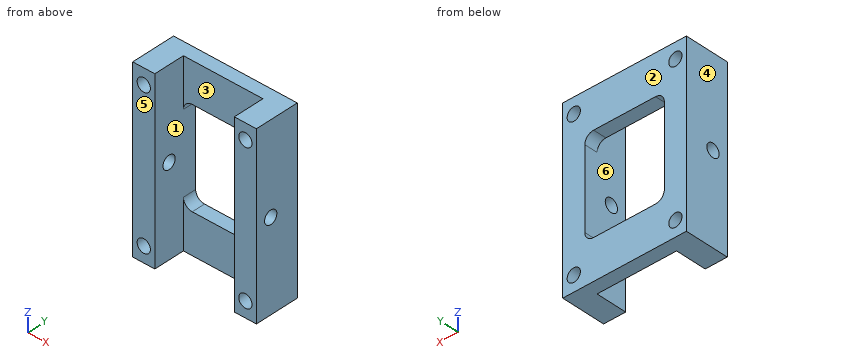
from build123d import *

# Parameters (mm, degrees)
EXTRUDE_1_DEPTH     = 40
SKETCH_2_R          = 1.5
CUT_EXTRUDE_1_DEPTH = 40
SKETCH_3_R          = 1.5
CUT_EXTRUDE_2_DEPTH = 40
SKETCH_5_W          = 18
SKETCH_5_H          = 22
CUT_EXTRUDE_3_DEPTH = 50.839743178
FILLET_3_R          = 2


with BuildPart() as part:
    # 草图1 → 凸台-拉伸1 (new body)
    with BuildSketch(Plane.XY):
        Polygon((0, 0), (0, 10), (28, 10), (28, 0), (23, 0), (23, 7), (5, 7), (5, 0), align=None)
    extrude(amount=EXTRUDE_1_DEPTH)

    # 草图2 → 切除-拉伸1 (cut)
    with BuildSketch(Plane(origin=(0, 10, 0), x_dir=(1, 0, 0), z_dir=(0, 1, 0))):
        with Locations(Location((2.5, -3.5, 0), (0, 0, 270))):
            Circle(SKETCH_2_R)
        with Locations(Location((2.5, -36.5, 0), (0, 0, 270))):
            Circle(SKETCH_2_R)
        with Locations(Location((25.5, -36.5, 0), (0, 0, 270))):
            Circle(SKETCH_2_R)
        with Locations(Location((25.5, -3.5, 0), (0, 0, 270))):
            Circle(SKETCH_2_R)
    extrude(amount=-CUT_EXTRUDE_1_DEPTH, mode=Mode.SUBTRACT)

    # 草图3 → 切除-拉伸2 (cut)
    with BuildSketch(Plane.ZY):
        with Locations((20, 3.5)):
            Circle(SKETCH_3_R)
    extrude(amount=-CUT_EXTRUDE_2_DEPTH, mode=Mode.SUBTRACT)

    # 草图5 → 切除-拉伸3 (cut, through all)
    with BuildSketch(Plane(origin=(0, 10, 0), x_dir=(1, 0, 0), z_dir=(0, 1, 0))):
        with Locations((14, -20)):
            Rectangle(SKETCH_5_W, SKETCH_5_H)
    extrude(amount=-CUT_EXTRUDE_3_DEPTH, mode=Mode.SUBTRACT)

    # 圆角3
    fillet_3_edges = [part.edges().sort_by_distance(p)[0] for p in [
        (23, 8.5, 31),
        (5, 8.5, 9),
        (5, 8.5, 31),
        (23, 8.5, 9),
    ]]
    fillet(fillet_3_edges, radius=FILLET_3_R)


solid = part.part
Verification items for the finished model (mm, model axes). Face numbers are marked on the shaded views. A direction names the side the tool comes from. Coordinates: 2 decimals unless noted, no trailing zeros. Order: outer loops, then holes, each group sorted by start corner. A loop starts at its lowest first (then second) coordinate and runs counter-clockwise, first axis right, second up. Notation, with made-up numbers: (-18.75, -38.5) -> (26.25, -38.5) arc R35 ccw to (26.25, -1.5) -> close; hole circle Ø5 at (45.25, 85). An arc over 180 degrees is marked (long way). Use CSV: the item, a comma, the result in double quotes. Start each with the question number.
Q1. Section check A-A, the plane x = 2.5. Record the cut outline in (y, z).
Q2. Draft check along X on the marked faces 4, 5 and 6. Enter one of: +X half, -X half, draft (parallel to the pull), parting line (faces both ways), or undercut.
Q3. Thickness scan on line 1 along X through (y, z) = (4.25, 3.5); line 2 along X through (y, z) = (5.75, 14); line 3 along Z through (x, y) = (14.25, 9). Record the ranges inside material, lowest first.
Q4. Section check C-C, the plane y = 3.5. Record the cut outline in (x, z), and give its area (3 significant figures).
Q5. Depth check by flat-ended pin: P1, Ø2.5, axis at x = 25.5, z = 3.5, coming from the +Y side; P2, Ø4, axis at y = 3.5, z = 20, coming from the -X side; P3, Ø5.5, axis at x = 11, z = 35.5, coming from the -Y side. Enter the tip coordinate at first touch or a pass-through.
Q6. Section check B-B, the plane y = 1.5. Record the cut outline in (x, z), and give its area (3 significant figures).
Q7. Section check D-D, the plane z = 20. Record the cut outline in (x, y), and give its area (3 significant figures).
Q8. Tool access check on the marked faces 1, 2 and 3. Record the directions out of +Z, -Z, +X, -X, +Y, -Y that give a thin tool (end or side, any length) a straight path to the whole face; none if there is none.
Returned:
1,outline,"(0, 0) -> (10, 0) -> (10, 2) -> (0, 2) -> close; (0, 5) -> (10, 5) -> (10, 35) -> (0, 35) -> close; (0, 38) -> (10, 38) -> (10, 40) -> (0, 40) -> close; hole circle Ø3 at (3.5, 20)"
2,face 4,"-X half"
2,face 5,"draft"
2,face 6,"undercut"
3,line 1,"x = 0 to 1, 4 to 5, 23 to 24, 27 to 28"
3,line 2,"x = 0 to 5, 23 to 28"
3,line 3,"z = 0 to 9, 31 to 40"
4,outline,"(0, 0) -> (5, 0) -> (5, 18.5) -> (0, 18.5) -> close; (0, 21.5) -> (5, 21.5) -> (5, 40) -> (0, 40) -> close; (23, 0) -> (28, 0) -> (28, 18.5) -> (23, 18.5) -> close; (23, 21.5) -> (28, 21.5) -> (28, 40) -> (23, 40) -> close; hole circle Ø3 at (2.5, 3.5); hole circle Ø3 at (2.5, 36.5); hole circle Ø3 at (25.5, 3.5); hole circle Ø3 at (25.5, 36.5)"
4,area,"342 mm^2"
5,P1,"passes through"
5,P2,"stops at x = 0"
5,P3,"stops at y = 7"
6,outline,"(0, 0) -> (5, 0) -> (5, 40) -> (0, 40) -> close; (23, 0) -> (28, 0) -> (28, 40) -> (23, 40) -> close; hole circle Ø3 at (2.5, 3.5); hole circle Ø3 at (2.5, 36.5); hole circle Ø3 at (25.5, 3.5); hole circle Ø3 at (25.5, 36.5)"
6,area,"372 mm^2"
7,outline,"(0, 0) -> (5, 0) -> (5, 2) -> (0, 2) -> close; (0, 5) -> (5, 5) -> (5, 10) -> (0, 10) -> close; (23, 0) -> (28, 0) -> (28, 2) -> (23, 2) -> close; (23, 5) -> (28, 5) -> (28, 10) -> (23, 10) -> close"
7,area,"70.0 mm^2"
8,face 1,"-Y"
8,face 2,"+Z, -Z, +X, -X, +Y"
8,face 3,"+Z, -Z, -Y"
